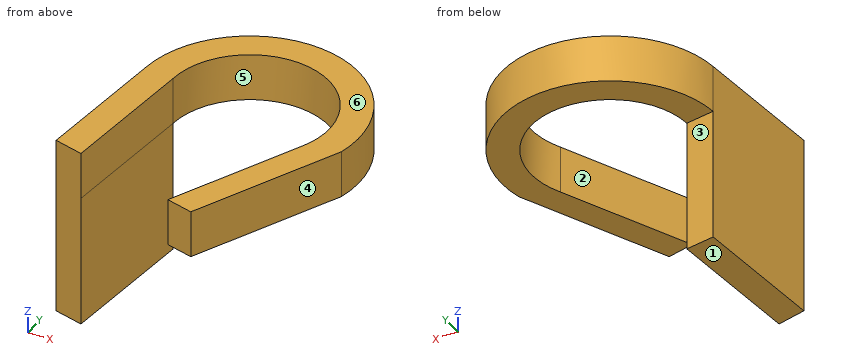
```python
from build123d import *

# Parameters (mm, degrees)
BOSS_EXTRUDE3_DEPTH = 10
BOSS_EXTRUDE4_DEPTH = 28


with BuildPart() as part:
    # Sketch1 → Boss-Extrude3 (new body)
    with BuildSketch(Plane.XY):
        with BuildLine():
            ThreePointArc((-16.733879942, 0.734685024), (4.365374373, 16.171147349), (14.830379862, -7.786034495))
            Line((14.830379862, -7.786034495), (1.98558973, -34.897127547))
            Line((1.98558973, -34.897127547), (7.660402975, -36.381590217))
            Line((7.660402975, -36.381590217), (22.375667903, -5.322545058))
            ThreePointArc((22.375667903, -5.322545058), (3.672252171, 22.704945805), (-22.912677541, 2.002300652))
            Line((-22.912677541, 2.002300652), (-25.690659105, -27.657354808))
            Line((-25.690659105, -27.657354808), (-19.543738844, -29.265314976))
            Line((-19.543738844, -29.265314976), (-16.733879942, 0.734685024))
        make_face()
    extrude(amount=BOSS_EXTRUDE3_DEPTH)

    # Sketch2 → Boss-Extrude4 (add)
    with BuildSketch(Plane(origin=(0, 0, 0), x_dir=(-1, 0, 0), z_dir=(0, 0, -1))):
        Polygon((22.912677541, 2.002300652), (16.720636216, 0.876084213), (19.543738844, -29.265314976), (25.690659105, -27.657354808), align=None)
    extrude(amount=BOSS_EXTRUDE4_DEPTH)


solid = part.part
```
Here's how the part is built. I have some questions about the finished solid (model axes, mm). Face numbers are marked on the shaded views. A direction names the side the tool comes from. Coordinates: 2 decimals unless noted, no trailing zeros. Loops run counter-clockwise (first coordinate to the right, second up) from the corner with the lowest first, then second, coordinate; pieces in that order, holes last. Notation, with made-up numbers: M 8.5,85.5 L 56.5,85.5 A16 cw 56.5,111.5 Z; hole C 6.5,-38 d8. An arc over 180 degrees is marked long. One line per item, written item: value.
1. Will these pins go through, and if not, where does the flat tip stop? pin 1 Ø1.5 at (y, z) = (5, 6) entering from +X; pin 2 Ø1 at (x, z) = (-16, -13.5) entering from -Y; pin 3 Ø12 at (y, z) = (-2, 1.5) entering from -X; pin 4 Ø2 at (y, z) = (-22, -24) entering from +X.
Geometry says:
pin 1: stops at x = 22.6
pin 2: passes through
pin 3: stops at x = -23.85
pin 4: stops at x = -18.77
2. Imagine slicing it at A-A (x = 11). List the corners of the cut face in (y, z) for me.
Geometry says:
outline: M -29.33,0 L -15.87,0 L -15.87,10 L -29.33,10 Z; M 12.63,0 L 20.2,0 L 20.2,10 L 12.63,10 Z
3. Imagine slicing it at C-C (z = 5.5). List the corners of the cut face in (x, y) for me.
Geometry says:
outline: M -25.69,-27.66 L -19.54,-29.27 L -16.73,0.73 A16.75 cw long 14.83,-7.79 L 1.99,-34.9 L 7.66,-36.38 L 22.38,-5.32 A23 ccw long -22.91,2 Z
4. On a 3-axis mill with a long thin cutter (end or side, diameter ignored), from which of +Z, -Z, +X, -X, +Y, -Y can I reach the whole of each face in a straight line? I mean the marked faces 1, 2 and 3. Say none if no direction works.
Geometry says:
face 1: -Z, +X, -X, +Y, -Y
face 2: +Z, -Z
face 3: -Z, +X, +Y
5. Imagine slicing it at D-D (y = 11). List the corners of the cut face in (x, z) for me.
Geometry says:
outline: M -20.2,0 L -12.63,0 L -12.63,10 L -20.2,10 Z; M 12.63,0 L 20.2,0 L 20.2,10 L 12.63,10 Z
6. Please list where these lines run through material, in increasing order: probe 1 along Z at (x, y) = (18.5, 4.5); probe 2 along Y at (x, z) = (0, 5); probe 3 along X at (y, z) = (0, 6).
Geometry says:
probe 1: z = 0 to 10
probe 2: y = 16.75 to 23
probe 3: x = -23.1 to -16.8, 16.75 to 23
7. Imagine slicing it at B-B (y = -22). List the corners of the cut face in (x, z) for me, and give its area (3 significant figures).
Geometry says:
outline: M -25.16,-28 L -18.86,-28 L -18.86,10 L -25.16,10 Z; M 8.1,0 L 14.47,0 L 14.47,10 L 8.1,10 Z
area: 303 mm2
8. Thinking about a two-plate mould opening in X: for the marked faces 4, 5 and 6, which applies, +X half, -X half, draft (parallel to the pull), parting line (faces both ways), or undercut?
Geometry says:
face 4: +X half
face 5: undercut
face 6: draft
